Drawing for the job (mm, zero at the part's lowest x, y, z). A direction names the side the tool comes from. Coordinates: 2 decimals unless noted, no trailing zeros. Write each loop counter-clockwise with the first axis right and the second up, starting at its lowest first coordinate (ties: lowest second). Pieces come first, ordered by that corner, then holes. Notation, with made-up numbers: M -14,-31 L 38,-31 A14 ccw 38,-15 Z; hole C 71.25,7 d10. An arc over 180 degrees is marked long. Put each result on its own line as item: value. Start each with the question number.
Q1. Drill centre lines: line 1 along Y through (x, z) = (12, 1.5); line 2 along Z through (x, y) = (14, 22.25); line 3 along Z through (x, y) = (10.75, 6.75). Where is each one in solid material? Low to high.
Q2. Cut at B-B (y = 12). Give the number of separate pieces and of enclosed holes in the cut face, then the cut area to 3 significant figures.
Q3. Drop flat-ended pins along their axis: pin 1 (2 mm diameter, centred on y = 18, z = 8.5, fed in from +X); pin 2 (1 mm diameter, centred on x = 11.5, y = 12, fed in from -Z); pin 3 (8 mm diameter, centred on y = 10, z = 16, fed in from +X); pin 4 (10 mm diameter, centred on x = 3, z = 14.5, fed in from +Y). Give the stop position or say it passes through.
Q4. Which spindle directions (+Z, -Z, +X, -X, +Y, -Y) get a long thin tool onto all of the face, cutting with end or side? Do the marked faces 4, 5 and 6. Say none if no direction does.
Q5. Pull direction X, two halves, no side cores. Call the marked faces 1, 2 and 3: pulls with the +X half, pulls with the -X half, needs draft (parallel to the pull), parting line crosses it, or undercut.
Q6. Cut at A-A (x = 12). Write the cut outline in (y, z).
Q7. Cut at C-C (z = 8.75). Write the cut outline in (x, y).
Q8. Cut at D-D (y = 20.75). Write the cut outline in (x, z).
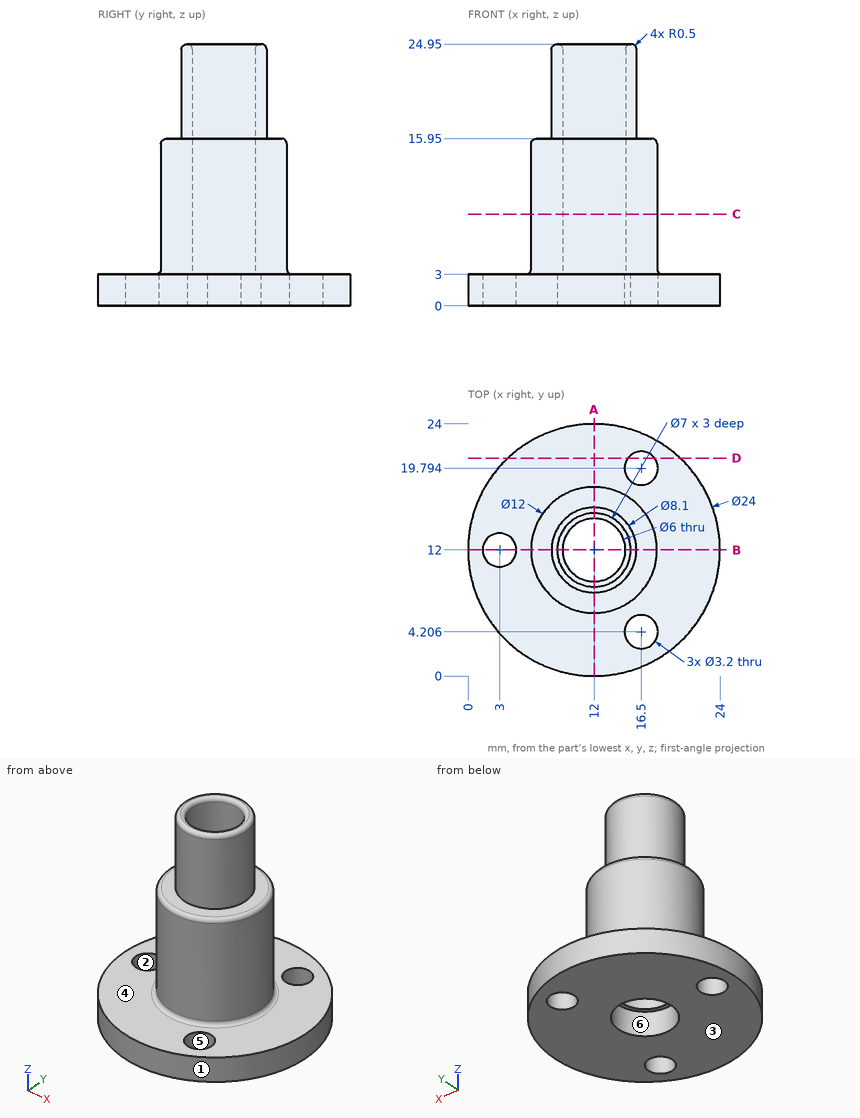
Computed values:
1. line 1: 0 to 8.5, 15.5 to 24
1. line 2: 0 to 3
1. line 3: 0 to 15.95
2. separate pieces: 3
2. enclosed holes: 0
2. area: 138 mm2
3. pin 1: x = 15.32
3. pin 2: through
3. pin 3: x = 18
3. pin 4: y = 16.47
4. face 4: +Z
4. face 5: +Z, -Z
4. face 6: -Z
5. face 1: parting line crosses it
5. face 2: undercut
5. face 3: needs draft
6. outline: M 0,0 L 8.5,0 L 8.5,3 L 9,3 L 9,24.45 A0.5 ccw 8.5,24.95 L 8.45,24.95 A0.5 ccw 7.95,24.45 L 7.95,15.95 L 6.5,15.95 A0.5 ccw 6,15.45 L 6,3.5 A0.5 cw 5.5,3 L 0,3 Z; M 15,3 L 15.5,3 L 15.5,0 L 24,0 L 24,3 L 18.5,3 A0.5 cw 18,3.5 L 18,15.45 A0.5 ccw 17.5,15.95 L 16.05,15.95 L 16.05,24.45 A0.5 ccw 15.55,24.95 L 15.5,24.95 A0.5 ccw 15,24.45 Z
7. outline: C 12,12 d12; hole C 12,12 d6
8. outline: M 3.79,0 L 15.22,0 L 15.22,3 L 3.79,3 Z; M 17.78,0 L 20.21,0 L 20.21,3 L 17.78,3 Z
